The model under review builds one solid part; all positions refer to its coordinate system, in mm. A direction names the side the tool comes from. Coordinates: 2 decimals unless noted, no trailing zeros. Order: outer loops, then holes, each group sorted by start corner. A loop starts at its lowest first (then second) coordinate and runs counter-clockwise, first axis right, second up. Notation, with made-up numbers: (-6, 33.25) -> (38, 33.25) arc R26 ccw to (38, 54.25) -> close; hole circle Ø10 at (15.5, 39.25). An arc over 180 degrees is marked (long way). Use one line per item in the form item = value.
Autodesk Inventor part; units mm, degrees
ref_plane "YZ Plane" through (0, 0, 0) normal (1, 0, 0) x (0, 1, 0)
ref_plane "XZ Plane" through (0, 0, 0) normal (0, 1, 0) x (-1, 0, 0)
ref_plane "XY Plane" through (0, 0, 0) normal (0, 0, 1) x (1, 0, 0)
sketch "Sketch1" plane through (0, 0, 0) normal (0, 1, 0) x (-1, 0, 0)
  line L0 (6.825, 0) -> (3.4125, -5.9106)
  line L1 (3.4125, -5.9106) -> (-3.4125, -5.9106)
  line L2 (-3.4125, -5.9106) -> (-6.825, 0)
  line L3 (-6.825, 0) -> (-3.4125, 5.9106)
  line L4 (-3.4125, 5.9106) -> (3.4125, 5.9106)
  line L5 (3.4125, 5.9106) -> (6.825, 0)
  point P0 (0, 0)
  point P1 (0, 0)
  dimension "d1" = 13.65
extrude "Extrusion1" add sketch "Sketch1" along normal blind 4.8
sketch "Sketch2" plane through (0, 4.8, 0) normal (0, 1, 0) x (1, 0, 0)
  circle A0 centre (0, 0) radius 5.5
  circle A1 centre (0, 0) radius 1.625
  line L0 (-1.1726, 1.125) -> (1.1726, 1.125)
  line L1 (0, -1.625) -> (0, 1.125)
  dimension "d4" = 11
  dimension "d5" = 3.25
  dimension "d56" = 2.75
extrude "Extrusion2" add sketch "Sketch2" along normal blind 14 contours A0 | L0 A1
sketch "Sketch7" plane through (-1.1726, 18.8, -1.125) normal (0, 0, 1) x (1, 0, 0)
  line L0 (0, 0) -> (2.3452, 0)
  line L1 (0, -14) -> (0, 0)
  line L2 (1.1726, 0) -> (1.1726, -3.5)
  circle A0 centre (1.1726, -3.5) radius 1
  point P0 (0, -0.5)
  point P1 (1.1726, -18.8)
  dimension "d33" = 3.5
  dimension "d34" = 2
hole "Hole1" at (0, 15.3, -1.125) direction (0, 0, -1) diameter 3.2 depth 8 tip angle 118
sketch "Sketch8" plane through (0, 0, 0) normal (0, -1, 0) x (1, 0, 0)
  circle A0 centre (0, 0) radius 1.5
  dimension "d42" = 3
hole "Hole2" at (0, 0, 0) direction (0, 1, 0) diameter 2.459 depth 7 tip angle 118
sketch "Sketch12" plane through (0, 18.8, 0) normal (0, 1, 0) x (1, 0, 0)
  line L0 (2.2, -3.8105) -> (-2.2, -3.8105)
  line L1 (-2.2, -3.8105) -> (-4.4, 0)
  line L2 (-4.4, 0) -> (-2.2, 3.8105)
  line L3 (-2.2, 3.8105) -> (2.2, 3.8105)
  line L4 (2.2, 3.8105) -> (4.4, 0)
  line L5 (4.4, 0) -> (2.2, -3.8105)
  line L6 (-1.1726, 1.125) -> (1.1726, 1.125)
  point P0 (0, 0)
  point P1 (0, 0)
  dimension "d64" = 4.4
  dimension "d69" = 7.621
extrude "Extrusion8" cut sketch "Sketch12" against normal blind 6
sketch "Sketch14" plane through (0, 18.8, 0) normal (0, 1, 0) x (1, 0, 0)
  circle A0 centre (0, 0) radius 5.5
  circle A1 centre (0, 0) radius 1.2282
extrude "Extrusion9" add sketch "Sketch14" along normal blind 1
Item 1: Tool access review of faces 1 (the face through (-0.481, 13.774, -4.667)), 2 (the face through (1, 4.8, 1)), 3 (the face through (0.471, 2.771, -1.136)): name each direction out of +Z, -Z, +X, -X, +Y, -Y from which nothing blocks a thin tool from reaching the whole face with its end or side.
Results found:
face_1 = -Z
face_2 = none
face_3 = -Y
Item 2: To check wall thickness, follow L1, parallel to X at y = 8.5, z = 0 (3 decimals); L2, parallel to Y at x = -1.5, z = 3.5; L3, parallel to Z at x = 0.25, y = 18.5. State the ranges of each line that lie inside material, in increasing order. Write a range as from..to.
Results found:
L1 = -5.5..-1.625, 1.625..5.5
L2 = 0..12.8, 18.8..19.8
L3 = -5.49..-3.81, 3.81..5.49
Item 3: Clearance check with flat-ended pins moving along their axes: pin 1 (1.9 mm diameter, centred on x = 0, y = 10, fed in from +Z); pin 2 (1 mm diameter, centred on x = -5, y = 14, fed in from +Z); pin 3 (5 mm diameter, centred on x = -1, y = 9.5, fed in from -Z); pin 4 (3 mm diameter, centred on x = 0, z = 0, fed in from -Y). State where each tip first meets the part, or that it passes through.
Results found:
pin_1 = 5.5
pin_2 = 3.16
pin_3 = -5.5
pin_4 = 0
Item 4: We need section A-A (x = 0). State how many separate pieces and enclosed holes the cut face has, plus the area to 3 significant figures.
Results found:
separate_pieces = 3
enclosed_holes = 0
area = 134 mm²
Item 5: We need section D-D (y = 15.3). Write out the cut boundary in (x, z).
Results found:
outline = (-4.4, 0) -> (-2.2, 3.81) -> (2.2, 3.81) -> (4.4, 0) -> (2.2, -3.81) -> (1.6, -3.81) -> (1.6, -5.26) arc R5.5 ccw (long way) to (-1.6, -5.26) -> (-1.6, -3.81) -> (-2.2, -3.81) -> close
Item 6: We need section B-B (y = 1.75). Write out the cut boundary in (x, z) (1 decimal), plus the area to 3 significant figures.
Results found:
outline = (-6.8, 0) -> (-3.4, -5.9) -> (3.4, -5.9) -> (6.8, 0) -> (3.4, 5.9) -> (-3.4, 5.9) -> close; hole circle Ø2.5 at (0, 0)
area = 116 mm²
Item 7: Draft analysis for pull direction Z (two halves, no side actions). For faces 4 (the face through (-5.143, 2.366, -2.914)), 5 (the face through (0, 16, 3.81)), 6 (the face through (2.957, 12.195, 4.638)), state which applies: released by +Z, released by -Z, zero draft, split by the parting line, or undercut.
Results found:
face_4 = released by -Z
face_5 = undercut
face_6 = split by the parting line
Item 8: We need section C-C (z = 3.5). Write out the cut boundary in (x, y), plus the area to 3 significant figures.
Results found:
outline = (-4.8, 0) -> (4.8, 0) -> (4.8, 4.8) -> (4.24, 4.8) -> (4.24, 19.8) -> (-4.24, 19.8) -> (-4.24, 4.8) -> (-4.8, 4.8) -> close; hole (-2.38, 12.8) -> (2.38, 12.8) -> (2.38, 18.8) -> (-2.38, 18.8) -> close
area = 145 mm²
